Check sheet for the modelled part. Datum: model origin and axes. Units: mm. A direction names the side the tool comes from. Coordinates: 2 decimals unless noted, no trailing zeros. Write each loop counter-clockwise with the first axis right and the second up, starting at its lowest first coordinate (ties: lowest second). Pieces come first, ordered by that corner, then holes. Notation, with made-up numbers: (70.5, -10) - (75.5, -10) arc R26 ccw to (75.5, 29) - close; hole circle Ø7 at (7, 82). An arc over 180 degrees is marked (long way). Answer as CSV lines item,"result". Start each with the question number.
from build123d import *

# Parameters (mm, degrees)
F1_DEPTH = 63.5
F2_DEPTH = 25.4
F3_DEPTH = 9.525
F0_W     = 25.4
F0_H     = 19.05
F4_DEPTH = 25.4
F6_R     = 6.35


# Not quite as in the source:
# - a feature names something its author has since deleted; it is built from what else it names


with BuildPart() as f1:
    # F0 (on Front) → F1 (new body, symmetric)
    with BuildSketch(Plane.XZ):
        Polygon((22.225, 9.525), (-41.275, 9.525), (-41.275, -9.525), (41.275, -9.525), (41.275, 9.525), align=None)
    extrude(amount=F1_DEPTH, both=True)

    # F0 (on Front) → F2 (join, symmetric)
    with BuildSketch(Plane.XZ):
        with BuildLine():
            Line((22.225, 27.0002), (22.225, 9.525))
            Line((22.225, 9.525), (41.275, 9.525))
            Line((41.275, 9.525), (41.275, 27.0002))
            ThreePointArc((41.275, 27.0002), (45.9246798487, 38.2255201513), (57.15, 42.8752))
            Line((57.15, 42.8752), (60.325, 42.8752))
            Line((60.325, 42.8752), (60.325, 61.9252))
            Line((60.325, 61.9252), (57.15, 61.9252))
            add(Edge.make_bspline(
                [(55.6853928695, 61.894476765), (56.1693943217, 61.9055488515), (56.6575757113, 61.9157865575), (57.15, 61.9252)],
                knots=[110.5437742754, 110.5437742754, 110.5437742754, 110.5437742754, 111.5045361635, 111.5045361635, 111.5045361635, 111.5045361635], degree=3))
            ThreePointArc((55.6853928695, 61.894476765), (31.9417966821, 51.1725418494), (22.225, 27.0002))
        make_face()
    extrude(amount=F2_DEPTH, both=True)

    # F0 (on Front) → F3 (join, symmetric)
    with BuildSketch(Plane.XZ):
        with BuildLine():
            add(Edge.make_bspline(
                [(-41.275, 9.525), (-0.3556397641, 48.3007017864), (-0.003064316, 60.620539654), (55.6853928695, 61.894476765)],
                knots=[0, 0, 0, 0, 110.5437742754, 110.5437742754, 110.5437742754, 110.5437742754], degree=3))
            Line((-41.275, 9.525), (22.225, 9.525))
            Line((22.225, 9.525), (22.225, 27.0002))
            ThreePointArc((22.225, 27.0002), (31.9417966821, 51.1725418494), (55.6853928695, 61.894476765))
        make_face()
    extrude(amount=F3_DEPTH, both=True)

    # F0 (on Front) → F4 (join, symmetric)
    with BuildSketch(Plane.XZ):
        with Locations((73.025, 52.4002)):
            Rectangle(F0_W, F0_H)
    extrude(amount=F4_DEPTH, both=True)

    # F0 (on Front) → F5 (revolve)
    with BuildSketch(Plane.XZ):
        Polygon((85.725, 66.675), (85.725, 61.9252), (85.725, 42.8752), (85.725, 38.1), (111.125, 38.1), (111.125, 66.675), align=None)
    revolve(axis=Axis((85.725, 0, 52.3875), (0, 0, -1)))

    # F6
    f6_edges = [f1.edges().sort_by_distance(p)[0] for p in [
        (41.275, -63.5, 0),
        (-41.275, -63.5, 0),
        (41.275, 63.5, 0),
        (-41.275, 63.5, 0),
    ]]
    fillet(f6_edges, radius=F6_R)


solid = f1.part
(1) Tool access check on faces 1 (the face through (32.2, 17.35, 51.44)), 2 (the face through (45.8, -0.4, 38.1)), 3 (the face through (60, 2, 42.875)), 4 (the face through (60, 2, 61.925)). Record the directions out of +Z, -Z, +X, -X, +Y, -Y that give a thin tool (end or side, any length) a straight path to the whole face; none if there is none.
(2) Cross-section at A-A on z = 2. Record the boundary of the cut face in (x, y) (3 decimals), plus the area to 3 significant figures.
(3) Material ranges on probe 1 along Z at (x, y) = (-33.5, -40) (3 decimals); probe 2 along X at (y, z) = (18, 13.5) (3 decimals), recorded low to high. Write a range as from..to.
(4) Cross-section at D-D on x = 91.5. Record the boundary of the cut face in (y, z) (3 decimals).
(5) Cross-section at B-B on x = 73. Record the boundary of the cut face in (y, z) (3 decimals), plus the area to 3 significant figures.
(6) Cross-section at C-C on y = 45. Record the boundary of the cut face in (x, z) (3 decimals), plus the area to 3 significant figures.
(7) Go/stop test with flat-tipped pins: P1, Ø2, axis at x = 32, z = 28.5, coming from the -Y side; P2, Ø16, axis at x = -13.5, y = 27, coming from the +Z side (3 decimals); P3, Ø1.5, axis at y = -7.5, z = 23.5, coming from the -X side. Record where each tip stops, or that it passes through.
Checked values:
1,face 1,"+Z, -X, +Y"
1,face 2,"-Z, +Y, -Y"
1,face 3,"-Z"
1,face 4,"+Z, -X"
2,outline,"(-41.275, -57.15) arc R6.35 ccw to (-34.925, -63.5) - (34.925, -63.5) arc R6.35 ccw to (41.275, -57.15) - (41.275, 57.15) arc R6.35 ccw to (34.925, 63.5) - (-34.925, 63.5) arc R6.35 ccw to (-41.275, 57.15) - close"
2,area,"10,400 mm^2"
3,probe 1,"-9.525..9.525"
3,probe 2,"22.225..41.275"
4,outline,"(-24.735, 38.1) - (24.735, 38.1) - (24.735, 66.675) - (-24.735, 66.675) - close"
5,outline,"(-25.4, 42.875) - (-21.983, 42.875) - (-21.983, 38.1) - (21.983, 38.1) - (21.983, 42.875) - (25.4, 42.875) - (25.4, 61.925) - (21.983, 61.925) - (21.983, 66.675) - (-21.983, 66.675) - (-21.983, 61.925) - (-25.4, 61.925) - close"
5,area,"1,390 mm^2"
6,outline,"(-41.275, -9.525) - (41.275, -9.525) - (41.275, 9.525) - (-41.275, 9.525) - close"
6,area,"1,570 mm^2"
7,P1,"y = -25.4"
7,P2,"z = 9.525"
7,P3,"x = -27.75"
